from build123d import *

# Parameters (mm, degrees)
SKETCH_1_W          = 3.5
SKETCH_1_H          = 12
EXTRUDE_1_DEPTH     = 12
SKETCH_2_R          = 0.5
EXTRUDE_2_DEPTH     = 3
CUT_EXTRUDE_1_DEPTH = 5
SKETCH_4_W          = 1.517225246
SKETCH_4_H          = 1.416076897
EXTRUDE_1_2_DEPTH   = 13.2


with BuildPart() as part:
    # 草图1 → Extrude 1 (new body)
    with BuildSketch(Plane(origin=(0, 0, 0), x_dir=(1, 0, 0), z_dir=(0, 1, 0))):
        Rectangle(SKETCH_1_W, SKETCH_1_H)
    extrude(amount=EXTRUDE_1_DEPTH)

    # 草图2 → 拉伸2 (add)
    with BuildSketch(Plane.XZ):
        with Locations(Location((0, 2.5, 0), (0, 0, 90))):
            Circle(SKETCH_2_R)
        with Locations(Location((0, -2.5, 0), (0, 0, 90))):
            Circle(SKETCH_2_R)
    extrude(amount=EXTRUDE_2_DEPTH)

    # 草图3 → 切除-拉伸1 (cut)
    with BuildSketch(Plane(origin=(1.75, 0, 0), x_dir=(0, 0, -1), z_dir=(1, 0, 0))):
        Polygon((-1.6, 12), (-6, 5), (-6, 12), align=None)
        Polygon((1.6, 12), (6, 7), (6, 12), align=None)
    extrude(amount=-CUT_EXTRUDE_1_DEPTH, mode=Mode.SUBTRACT)

    # 草图4 → Extrude 1 2 (add)
    with BuildSketch(Plane.XZ):
        with Locations((0, 2.950160203)):
            Rectangle(SKETCH_4_W, SKETCH_4_H)
    extrude(amount=-EXTRUDE_1_2_DEPTH)


solid = part.part
The model under review builds one solid part; all positions refer to its coordinate system, in mm. A direction names the side the tool comes from. Coordinates: 2 decimals unless noted, no trailing zeros. Write each loop counter-clockwise with the first axis right and the second up, starting at its lowest first coordinate (ties: lowest second). Pieces come first, ordered by that corner, then holes. Notation, with made-up numbers: M 6,85.25 L 21,85.25 A18 cw 21,96.25 Z; hole C -37.75,-12 d1. An arc over 180 degrees is marked long. Put each result on its own line as item: value.
1) Wall thickness on probe 1 along Y at (x, z) = (1.1, -0.25); probe 2 along Y at (x, z) = (-0.4, 3.5); probe 3 along Z at (x, y) = (0.4, -0.5): over which ranges is each line inside the solid? List them lowest first. Write a range as [from, to].
Computed:
probe 1: y = [0, 12]
probe 2: y = [0, 13.2]
probe 3: z = [-2.8, -2.2], [2.2, 2.8]
2) Draft analysis for pull direction Z (two halves, no side actions). For faces 5 (the flat face through (0, 13.2, 3)), 6 (the flat face through (0, 9.5, -3.8)), 7 (the cylindrical face through (0, -1, 2)), 8 (the flat face through (0, 2, 6)), state which applies: released by +Z, released by -Z, zero draft, split by the parting line, or undercut.
Computed:
face 5: zero draft
face 6: released by -Z
face 7: undercut
face 8: released by +Z
3) Clearance check with flat-ended pins moving along their axes: pin 1 Ø1.7 at (x, y) = (0.5, 11) entering from +Z; pin 2 Ø1.2 at (x, y) = (0, 12.5) entering from -Z; pin 3 Ø1 at (x, z) = (0, 1) entering from -Y. State where each tip first meets the part, or that it passes through.
Computed:
pin 1: stops at z = 3.66
pin 2: stops at z = -1.69
pin 3: stops at y = 0
4) Add section A-A on x = 0. Give the boundary of the cut face in (y, z), then the cut area to 3 significant figures.
Computed:
outline: M -3,-3 L 0,-3 L 0,-6 L 7,-6 L 12,-1.6 L 12,1.6 L 10.98,2.24 L 13.2,2.24 L 13.2,3.66 L 8.73,3.66 L 5,6 L 0,6 L 0,3 L -3,3 L -3,2 L 0,2 L 0,-2 L -3,-2 Z
area: 128 mm2
5) For faces 1 (the flat face through (0, 11, 3.658)), 2 (the cylindrical face through (0, -1, -3)), 3 (the flat face through (-0.759, 11, 3)), 4 (the flat face through (0.759, 11, 3)), list the 3-axis set-ups (+Z, -Z, +X, -X, +Y, -Y) from which the entire face can be reached by the end or side of a thin tool; tool diameter is ignored.
Computed:
face 1: +Z, +X, -X, +Y
face 2: -Y
face 3: +Z, -X, +Y
face 4: +Z, +X, +Y
6) Add section B-B on z = 2.5. Give the boundary of the cut face in (x, y), then the cut area to 3 significant figures.
Computed:
outline: M -1.75,0 L -0.5,0 L -0.5,-3 L 0.5,-3 L 0.5,0 L 1.75,0 L 1.75,10.57 L 0.76,10.57 L 0.76,13.2 L -0.76,13.2 L -0.76,10.57 L -1.75,10.57 Z
area: 44.0 mm2
7) Add section C-C on y = 5.75. Give the boundary of the cut face in (x, z), then the cut area to 4 significant figures.
Computed:
outline: M -1.75,-6 L 1.75,-6 L 1.75,5.53 L -1.75,5.53 Z
area: 40.35 mm2
8) Add section D-D on z = 1. Give the boundary of the cut face in (x, y).
Computed:
outline: M -1.75,0 L 1.75,0 L 1.75,12 L -1.75,12 Z
